The model under review builds one solid part; all positions refer to its coordinate system, in mm. Round coordinates to 2 decimals unless told otherwise and drop trailing zeros. Order: outer loops, then holes, each group sorted by start corner. A loop starts at its lowest first (then second) coordinate and runs counter-clockwise, first axis right, second up.
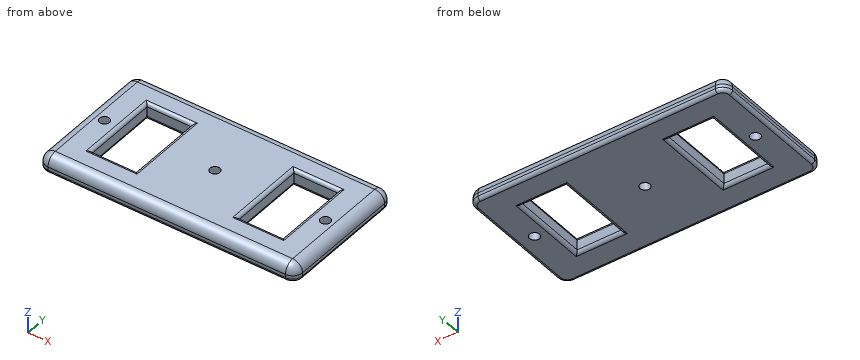
```python
from build123d import *

# Parameters (mm, degrees)
F0_R     = 1.5
F0_W     = 13.5
F0_H     = 23
F1_DEPTH = 5
F2_R     = 3
F3_R     = 1
F4_R     = 1


with BuildPart() as f1:
    # F0 (on Top) → F1 (new body)
    with BuildSketch(Plane.XY):
        Polygon((0, 20), (-39, 20), (-39, -20), (39, -20), (39, 0), (39, 20), align=None)
        with Locations((-33.5, 0)):
            Circle(F0_R, mode=Mode.SUBTRACT)
        with Locations((-22.25, 0)):
            Rectangle(F0_W, F0_H, mode=Mode.SUBTRACT)
        Circle(F0_R, mode=Mode.SUBTRACT)
        Polygon((15.5, 11.5), (29, 11.5), (29, 0), (29, -11.5), (15.5, -11.5), align=None, mode=Mode.SUBTRACT)
        with Locations((33.5, 0)):
            Circle(F0_R, mode=Mode.SUBTRACT)
    extrude(amount=F1_DEPTH)

    # F2
    f2_edges = [f1.edges().sort_by_distance(p)[0] for p in [
        (0, 20, 5),
        (-39, 0, 5),
        (0, -20, 5),
        (39, 0, 5),
        (-39, -20, 2.5),
        (-39, 20, 2.5),
        (39, 20, 2.5),
        (39, -20, 2.5),
    ]]
    fillet(f2_edges, radius=F2_R)

    # F3
    f3_edges = [f1.edges().sort_by_distance(p)[0] for p in [
        (0, -20, 0),
    ]]
    fillet(f3_edges, radius=F3_R)

    # F4
    f4_edges = [f1.edges().sort_by_distance(p)[0] for p in [
        (-22.25, -11.5, 5),
        (-15.5, 0, 5),
        (-22.25, 11.5, 5),
        (-29, 0, 5),
        (15.5, 0, 5),
        (22.25, 11.5, 5),
        (29, 0, 5),
        (22.25, -11.5, 5),
        (-29, 0, 0),
        (-15.5, 0, 0),
        (-22.25, 11.5, 0),
        (-22.25, -11.5, 0),
        (22.25, -11.5, 0),
        (29, 0, 0),
        (22.25, 11.5, 0),
        (15.5, 0, 0),
    ]]
    fillet(f4_edges, radius=F4_R)


solid = f1.part
```
(1) Insertion check: pin 1 (1.5 mm diameter, centred on x = -21.5, z = 3, fed in from -Y); pin 2 (1.5 mm diameter, centred on x = 10, z = 3.5, fed in from +Y); pin 3 (2 mm diameter, centred on x = 16, y = 8.5, fed in from +Z); pin 4 (2.5 mm diameter, centred on x = 0, y = 0, fed in from +Z). Each pin has a flat end and moves straight along its axis. Give the tip position at first contact, or say it passes through.
Data:
pin 1: stops at y = -19.99
pin 2: stops at y = 19.9
pin 3: stops at z = 4.87
pin 4: passes through
(2) To check wall thickness, follow probe 1 along X at (y, z) = (-4, 1.1); probe 2 along Y at (x, z) = (24, 1.8); probe 3 along X at (y, z) = (-10, 0.25). State the ranges of each line that lie inside material, in increasing order.
Data:
probe 1: x = -39 to -29, -15.5 to 15.5, 29 to 39
probe 2: y = -20 to -11.5, 11.5 to 20
probe 3: x = -38.66 to -29.34, -15.16 to 15.16, 29.34 to 38.66
(3) Consider section A-A (x = -33.5). Write out the cut boundary in (y, z).
Data:
outline: (-20, 1) arc R1 ccw to (-19, 0) - (-1.5, 0) - (-1.5, 5) - (-17, 5) arc R3 ccw to (-20, 2) - close; (1.5, 0) - (19, 0) arc R1 ccw to (20, 1) - (20, 2) arc R3 ccw to (17, 5) - (1.5, 5) - close
(4) Consider section B-B (y = -4). Write out the cut boundary in (x, z).
Data:
outline: (-39, 1) arc R1 ccw to (-38, 0) - (-30, 0) arc R1 ccw to (-29, 1) - (-29, 4) arc R1 ccw to (-30, 5) - (-36, 5) arc R3 ccw to (-39, 2) - close; (-15.5, 1) arc R1 ccw to (-14.5, 0) - (14.5, 0) arc R1 ccw to (15.5, 1) - (15.5, 4) arc R1 ccw to (14.5, 5) - (-14.5, 5) arc R1 ccw to (-15.5, 4) - close; (29, 1) arc R1 ccw to (30, 0) - (38, 0) arc R1 ccw to (39, 1) - (39, 2) arc R3 ccw to (36, 5) - (30, 5) arc R1 ccw to (29, 4) - close
(5) Consider section D-D (y = 0). State how many separate pieces and enclosed holes the cut face has, and give its area (3 significant figures).
Data:
separate pieces: 6
enclosed holes: 0
area: 204 mm2
(6) Consider section C-C (x = -3.5). Write out the cut boundary in (y, z).
Data:
outline: (-20, 1) arc R1 ccw to (-19, 0) - (19, 0) arc R1 ccw to (20, 1) - (20, 2) arc R3 ccw to (17, 5) - (-17, 5) arc R3 ccw to (-20, 2) - close
